from build123d import *

# Parameters (mm, degrees)
SKETCH1_W           = 13.75
SKETCH1_H           = 13.75
BOSS_EXTRUDE1_DEPTH = 25
SKETCH3_R           = 3.75
CUT_EXTRUDE2_DEPTH  = 30.348392205
SKETCH4_R           = 6.55
CUT_EXTRUDE3_DEPTH  = 5
SKETCH8_R           = 1.4
CUT_EXTRUDE6_DEPTH  = 30.348392205
SKETCH9_R           = 1.5
CUT_EXTRUDE7_DEPTH  = 27.824079667
CHAMFER1_SIZE       = 1
FILLET2_R           = 1


with BuildPart() as part:
    # Sketch1 → Boss-Extrude1 (new body)
    with BuildSketch(Plane.XY):
        Rectangle(SKETCH1_W, SKETCH1_H)
    extrude(amount=BOSS_EXTRUDE1_DEPTH)

    # Sketch3 → Cut-Extrude2 (cut, through all)
    with BuildSketch(Plane(origin=(0, 6.875, 0), x_dir=(1, 0, 0), z_dir=(0, 1, 0))):
        with Locations(Location((0, -9.5, 0), (0, 0, 270))):
            Circle(SKETCH3_R)
    extrude(amount=-CUT_EXTRUDE2_DEPTH, mode=Mode.SUBTRACT)

    # Sketch4 → Cut-Extrude3 (cut)
    with BuildSketch(Plane(origin=(0, 6.875, 0), x_dir=(1, 0, 0), z_dir=(0, 1, 0))):
        with Locations(Location((0, -9.5, 0), (0, 0, 270))):
            Circle(SKETCH4_R)
    cut_extrude3 = extrude(amount=-CUT_EXTRUDE3_DEPTH, mode=Mode.SUBTRACT)

    # Mirror4: Cut-Extrude3 across plane
    add(cut_extrude3.mirror(Plane.ZX), mode=Mode.SUBTRACT)

    # Sketch8 → Cut-Extrude6 (cut, through all)
    with BuildSketch(Plane(origin=(0, 6.875, 0), x_dir=(1, 0, 0), z_dir=(0, 1, 0))):
        with Locations(Location((0, -20.5, 0), (0, 0, 270))):
            Circle(SKETCH8_R)
    extrude(amount=-CUT_EXTRUDE6_DEPTH, mode=Mode.SUBTRACT)

    # Sketch9 → Cut-Extrude7 (cut, through all)
    with BuildSketch(Plane(origin=(0, 0, 0), x_dir=(-1, 0, 0), z_dir=(0, 0, -1))):
        with Locations((-4, 0)):
            Circle(SKETCH9_R)
    cut_extrude7 = extrude(amount=-CUT_EXTRUDE7_DEPTH, mode=Mode.SUBTRACT)

    # Mirror5: Cut-Extrude7 across plane
    add(cut_extrude7.mirror(Plane(origin=(0, 0, 0), x_dir=(0, 0, 1), z_dir=(1, 0, 0))), mode=Mode.SUBTRACT)

    # Chamfer1
    chamfer1_edges = [part.edges().sort_by_distance(p)[0] for p in [
        (0, -6.875, 19.1),
        (0, 6.875, 19.1),
    ]]
    chamfer(chamfer1_edges, length=CHAMFER1_SIZE)

    # Fillet2
    # the kernel refuses this fillet: 1 mm, written as the material it takes off along each edge
    with BuildSketch(Plane(origin=(-5.875, 5.875, 24), x_dir=(-1, 0, 0), z_dir=(0, 1, 0))) as fillet2_piece_1_section:
        Polygon((0, 0), (FILLET2_R, 0), (FILLET2_R, FILLET2_R), (0, FILLET2_R), align=None)
    fillet2_piece_1 = extrude(amount=FILLET2_R, mode=Mode.PRIVATE)
    fillet2_piece_1 = fillet2_piece_1 - Plane(origin=(-5.875, 5.875, 24), x_dir=(0.7071067811865475, 0, -0.7071067811865475), z_dir=(0, 1, 0)) * Sphere(FILLET2_R, mode=Mode.PRIVATE)
    add(fillet2_piece_1, mode=Mode.SUBTRACT)
    with BuildSketch(Plane(origin=(5.875, 5.875, 24), x_dir=(0, 0, 1), z_dir=(0, 1, 0))) as fillet2_piece_2_section:
        Polygon((0, 0), (FILLET2_R, 0), (FILLET2_R, FILLET2_R), (0, FILLET2_R), align=None)
    fillet2_piece_2 = extrude(amount=FILLET2_R, mode=Mode.PRIVATE)
    fillet2_piece_2 = fillet2_piece_2 - Plane(origin=(5.875, 5.875, 24), x_dir=(-0.7071067811865475, 0, -0.7071067811865475), z_dir=(0, 1, 0)) * Sphere(FILLET2_R, mode=Mode.PRIVATE)
    add(fillet2_piece_2, mode=Mode.SUBTRACT)
    with BuildSketch(Plane(origin=(-5.875, -5.875, 1), x_dir=(-1, 0, 0), z_dir=(0, -1, 0))) as fillet2_piece_3_section:
        Polygon((0, 0), (FILLET2_R, 0), (FILLET2_R, FILLET2_R), (0, FILLET2_R), align=None)
    fillet2_piece_3 = extrude(amount=FILLET2_R, mode=Mode.PRIVATE)
    fillet2_piece_3 = fillet2_piece_3 - Plane(origin=(-5.875, -5.875, 1), x_dir=(0.7071067811865475, 0, 0.7071067811865475), z_dir=(0, -1, 0)) * Sphere(FILLET2_R, mode=Mode.PRIVATE)
    add(fillet2_piece_3, mode=Mode.SUBTRACT)
    with BuildSketch(Plane(origin=(5.875, -5.875, 1), x_dir=(0, 0, -1), z_dir=(0, -1, 0))) as fillet2_piece_4_section:
        Polygon((0, 0), (FILLET2_R, 0), (FILLET2_R, FILLET2_R), (0, FILLET2_R), align=None)
    fillet2_piece_4 = extrude(amount=FILLET2_R, mode=Mode.PRIVATE)
    fillet2_piece_4 = fillet2_piece_4 - Plane(origin=(5.875, -5.875, 1), x_dir=(-0.7071067811865475, 0, 0.7071067811865475), z_dir=(0, -1, 0)) * Sphere(FILLET2_R, mode=Mode.PRIVATE)
    add(fillet2_piece_4, mode=Mode.SUBTRACT)
    with BuildSketch(Plane(origin=(-5.875, 5.875, 1), x_dir=(-1, 0, 0), z_dir=(0, 1, 0))) as fillet2_piece_5_section:
        Polygon((0, 0), (FILLET2_R, 0), (FILLET2_R, -FILLET2_R), (0, -FILLET2_R), align=None)
    fillet2_piece_5 = extrude(amount=FILLET2_R, mode=Mode.PRIVATE)
    fillet2_piece_5 = fillet2_piece_5 - Plane(origin=(-5.875, 5.875, 1), x_dir=(0.7071067811865475, 0, 0.7071067811865475), z_dir=(0, 1, 0)) * Sphere(FILLET2_R, mode=Mode.PRIVATE)
    add(fillet2_piece_5, mode=Mode.SUBTRACT)
    with BuildSketch(Plane(origin=(5.875, 5.875, 1), x_dir=(0, 0, -1), z_dir=(0, 1, 0))) as fillet2_piece_6_section:
        Polygon((0, 0), (FILLET2_R, 0), (FILLET2_R, -FILLET2_R), (0, -FILLET2_R), align=None)
    fillet2_piece_6 = extrude(amount=FILLET2_R, mode=Mode.PRIVATE)
    fillet2_piece_6 = fillet2_piece_6 - Plane(origin=(5.875, 5.875, 1), x_dir=(-0.7071067811865475, 0, 0.7071067811865475), z_dir=(0, 1, 0)) * Sphere(FILLET2_R, mode=Mode.PRIVATE)
    add(fillet2_piece_6, mode=Mode.SUBTRACT)
    with BuildSketch(Plane(origin=(-6.875, 5.875, 25), x_dir=(0, 0, -1), z_dir=(0, -1, 0))) as fillet2_piece_7:
        with BuildLine():
            CenterArc((FILLET2_R, FILLET2_R), FILLET2_R, 180, 90)
            Line((0, FILLET2_R), (0, 0))
            Line((0, 0), (FILLET2_R, 0))
        make_face()
    extrude(amount=15.25, mode=Mode.SUBTRACT)
    with BuildSketch(Plane(origin=(6.875, -9.375, 25), x_dir=(-1, 0, 0), z_dir=(0, 1, 0))) as fillet2_piece_8:
        with BuildLine():
            CenterArc((FILLET2_R, -FILLET2_R), FILLET2_R, 90, 90)
            Line((0, -FILLET2_R), (0, 0))
            Line((0, 0), (FILLET2_R, 0))
        make_face()
    extrude(amount=15.25, mode=Mode.SUBTRACT)
    with BuildSketch(Plane(origin=(-5.875, -6.875, 0), x_dir=(0, 0, 1), z_dir=(1, 0, 0)), Plane(origin=(-6.875, 5.875, 0), x_dir=(0, 0, 1), z_dir=(0, -1, 0)), Plane(origin=(5.875, 6.875, 25), x_dir=(0, -1, 0), z_dir=(-1, 0, 0))) as fillet2_piece_9:
        with BuildLine():
            CenterArc((FILLET2_R, -FILLET2_R), FILLET2_R, 90, 90)
            Line((0, -FILLET2_R), (0, 0))
            Line((0, 0), (FILLET2_R, 0))
        make_face()
    extrude(amount=11.75, mode=Mode.SUBTRACT)
    with BuildSketch(Plane(origin=(5.875, 6.875, 0), x_dir=(0, -1, 0), z_dir=(-1, 0, 0)), Plane(origin=(6.875, -5.875, 0), x_dir=(-1, 0, 0), z_dir=(0, 1, 0))) as fillet2_piece_10:
        with BuildLine():
            CenterArc((FILLET2_R, FILLET2_R), FILLET2_R, 180, 90)
            Line((0, FILLET2_R), (0, 0))
            Line((0, 0), (FILLET2_R, 0))
        make_face()
    extrude(amount=11.75, mode=Mode.SUBTRACT)
    with BuildSketch(Plane(origin=(6.875, -6.875, 1), x_dir=(-1, 0, 0), z_dir=(0, 0, 1))) as fillet2_piece_11:
        with BuildLine():
            CenterArc((FILLET2_R, -FILLET2_R), FILLET2_R, 90, 90)
            Line((0, -FILLET2_R), (0, 0))
            Line((0, 0), (FILLET2_R, 0))
        make_face()
    extrude(amount=26.5, mode=Mode.SUBTRACT)
    with BuildSketch(Plane(origin=(-6.875, -6.875, 1), x_dir=(1, 0, 0), z_dir=(0, 0, 1))) as fillet2_piece_12:
        with BuildLine():
            CenterArc((FILLET2_R, FILLET2_R), FILLET2_R, 180, 90)
            Line((0, FILLET2_R), (0, 0))
            Line((0, 0), (FILLET2_R, 0))
        make_face()
    extrude(amount=26.5, mode=Mode.SUBTRACT)
    with BuildSketch(Plane(origin=(-6.875, 6.875, 1), x_dir=(0, -1, 0), z_dir=(0, 0, 1))) as fillet2_piece_13:
        with BuildLine():
            CenterArc((FILLET2_R, FILLET2_R), FILLET2_R, 180, 90)
            Line((0, FILLET2_R), (0, 0))
            Line((0, 0), (FILLET2_R, 0))
        make_face()
    extrude(amount=23, mode=Mode.SUBTRACT)
    with BuildSketch(Plane(origin=(6.875, 6.875, 1), x_dir=(0, -1, 0), z_dir=(0, 0, 1))) as fillet2_piece_14:
        with BuildLine():
            CenterArc((FILLET2_R, -FILLET2_R), FILLET2_R, 90, 90)
            Line((0, -FILLET2_R), (0, 0))
            Line((0, 0), (FILLET2_R, 0))
        make_face()
    extrude(amount=23, mode=Mode.SUBTRACT)


solid = part.part
Can you work these out from the model? Positions are in its coordinate system, mm. A direction names the side the tool comes from. Round coordinates to 2 decimals unless told otherwise and drop trailing zeros. Order: outer loops, then holes, each group sorted by start corner. A loop starts at its lowest first (then second) coordinate and runs counter-clockwise, first axis right, second up. Notation, with made-up numbers: M 85,-34.5 L 114,-34.5 A23 ccw 114,-24.5 Z; hole C 69.25,82.5 d5. An arc over 180 degrees is marked long. Use a Markdown table: item, result.
1) I'm going to push flat-ended pins straight in: P1, Ø1.7, axis at x = 0, z = 20.5, coming from the +Y side; P2, Ø1, axis at x = -1.5, z = 12.5, coming from the -Y side (3 decimals); P3, Ø4, axis at x = 2.5, z = 7, coming from the +Y side (3 decimals). Where does each tip first touch, or does it pass through?
Geometry says:
| item | result |
|---|---|
| P1 | passes through |
| P2 | stops at y = -1.875 |
| P3 | stops at y = 1.875 |
2) If we mould it in two halves opening along Z, with no side actions, what happens to faces 4 (the face through (0.08, 6.59, 0.3)), 5 (the face through (-0.54, 0.08, 21.79)), 6 (the face through (6.574, -6.59, 12.832))? For each: +Z half, -Z half, draft (parallel to the pull), parting line (faces both ways), or undercut.
Geometry says:
| item | result |
|---|---|
| face 4 | -Z half |
| face 5 | undercut |
| face 6 | draft |
3) Imagine slicing it at B-B (z = 20.5). List the corners of the cut face in (x, y) for me (3 decimals), then the cut area to 3 significant figures.
Geometry says:
| item | result |
|---|---|
| outline | M -6.875,-5.875 A1 ccw -5.875,-6.875 L -2.4,-6.875 L -1.4,-5.875 L -1.4,5.875 L -2.4,6.875 L -5.875,6.875 A1 ccw -6.875,5.875 Z; M 1.4,-5.875 L 2.4,-6.875 L 5.875,-6.875 A1 ccw 6.875,-5.875 L 6.875,5.875 A1 ccw 5.875,6.875 L 2.4,6.875 L 1.4,5.875 Z; hole C -4,0 d3; hole C 4,0 d3 |
| area | 134 mm² |
4) Imagine slicing it at A-A (x = 0). List the corners of the cut face in (y, z) for me (3 decimals), then the cut area to 3 significant figures.
Geometry says:
| item | result |
|---|---|
| outline | M -6.875,1 A1 ccw -5.875,0 L 5.875,0 A1 ccw 6.875,1 L 6.875,2.95 L 1.875,2.95 L 1.875,5.75 L -1.875,5.75 L -1.875,2.95 L -6.875,2.95 Z; M -6.875,16.05 L -1.875,16.05 L -1.875,13.25 L 1.875,13.25 L 1.875,16.05 L 6.875,16.05 L 6.875,18.1 L 5.875,19.1 L -5.875,19.1 L -6.875,18.1 Z; M -6.875,22.9 L -5.875,21.9 L 5.875,21.9 L 6.875,22.9 L 6.875,24 A1 ccw 5.875,25 L -6.875,25 Z |
| area | 143 mm² |
5) If I drill on line 1 along X through (y, z) = (-1, 2.25) (3 decimals); line 2 along X through (y, z) = (-0.75, 5.5) (3 decimals); line 3 along Y through (x, z) = (4.25, 10.75) (3 decimals), over which ranges is the centre line in solid material (lowest first)?
Geometry says:
| item | result |
|---|---|
| line 1 | x = -6.875 to -5.118, -2.882 to 2.882, 5.118 to 6.875 |
| line 2 | x = -6.875 to -5.299, -2.701 to 2.701, 5.299 to 6.875 |
| line 3 | y = -1.875 to -1.479, 1.479 to 1.875 |
6) Imagine slicing it at C-C (y = -0.5). List the corners of the cut face in (x, z) for me (3 decimals).
Geometry says:
| item | result |
|---|---|
| outline | M -6.875,1 A1 ccw -5.875,0 L -5.414,0 L -5.414,25 L -5.875,25 A1 ccw -6.875,24 Z; M -2.586,0 L 2.586,0 L 2.586,6.784 A3.75 cw -2.586,6.784 Z; M -2.586,12.216 A3.75 cw 2.586,12.216 L 2.586,25 L -2.586,25 Z; M 5.414,0 L 5.875,0 A1 ccw 6.875,1 L 6.875,24 A1 ccw 5.875,25 L 5.414,25 Z; hole C 0,20.5 d2.8 |
7) Imagine slicing it at D-D (y = -5.25). List the corners of the cut face in (x, z) for me (3 decimals).
Geometry says:
| item | result |
|---|---|
| outline | M -6.875,1 A1 ccw -5.875,0 L 5.875,0 A1 ccw 6.875,1 L 6.875,24 A1 ccw 5.875,25 L -5.875,25 A1 ccw -6.875,24 Z; hole C 0,9.5 d13.1; hole C 0,20.5 d2.8 |
8) On a 3-axis mill with a long thin cutter (end or side, diameter ignored), from which of +Z, -Z, +X, -X, +Y, -Y can I reach the whole of each face in a straight line? I mean faces 1 (the face through (-3, -1.875, 12)), 2 (the face through (-6.875, 0, 12)), 3 (the face through (1.967, 4.41, 15.748)). Say none if no direction works.
Geometry says:
| item | result |
|---|---|
| face 1 | -Y |
| face 2 | +Z, -Z, -X, +Y, -Y |
| face 3 | +Y |
